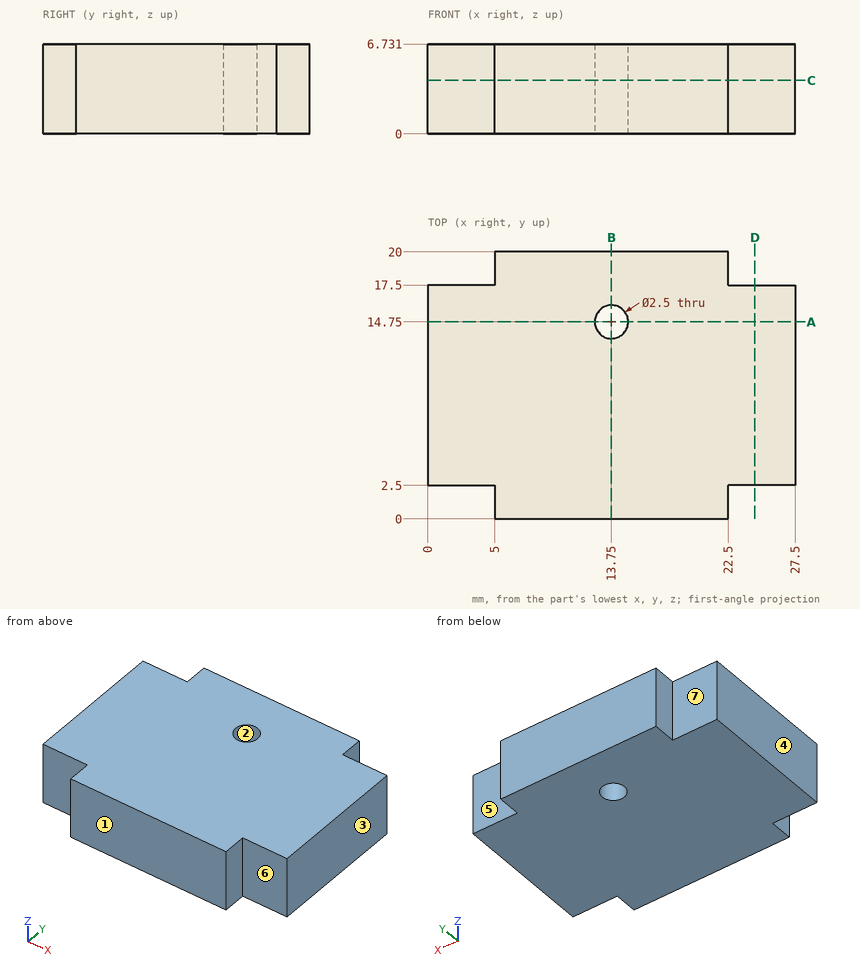
Geometry: see drawing. Coordinates: mm, zero at the bounding-box minimum. A direction names the side the tool comes from. Give positions to 0.01 mm unless a question says otherwise; leave off trailing zeros. Order: outer loops, then holes, each group sorted by start corner. A loop starts at its lowest first (then second) coordinate and runs counter-clockwise, first axis right, second up. Notation, with made-up numbers: M 86.5,-20.75 L 126.5,-20.75 A25 cw 126.5,15.25 Z; hole C -32.5,60.25 d10. An arc over 180 degrees is marked long. Answer as a JSON object with one key per item and string values.
1. First-contact query: P1, Ø1.5, axis at x = 24, z = 4, coming from the -Y side; P2, Ø2.5, axis at x = 1.5, z = 3.5, coming from the +Y side; P3, Ø2, axis at y = 19, z = 2.5, coming from the -X side; P4, Ø2, axis at x = 13.75, y = 14.75, coming from the -Z side. Flat tips, straight axial feed; report the tip coordinate or a pass-through.
Result sheet:
{"P1": "y = 2.5", "P2": "y = 17.5", "P3": "x = 5", "P4": "through"}
2. Reachability of the marked faces 5, 6 and 7 from +Z, -Z, +X, -X, +Y, -Y: full face, straight path, thin tool, end or side. Return the list, or none.
Result sheet:
{"face 5": "+Z, -Z, +X, +Y", "face 6": "+Z, -Z, +X, -Y", "face 7": "+Z, -Z, -X, +Y"}
3. Ray query, line 1 (Y direction, x = 13.75, z = 2.5); line 2 (Y direction, x = 14.75, z = 2.5); line 3 (X direction, y = 1.5, z = 3.75). Return the intervals inside material, ascending. Write a range as [from, to].
Result sheet:
{"line 1": "[0, 13.5], [16, 20]", "line 2": "[0, 14], [15.5, 20]", "line 3": "[5, 22.5]"}
4. Pull-direction query (X, two-part tool) for the marked faces 1, 2, 3 and 4; classes: +X half, -X half, draft (parallel to the pull), parting line (faces both ways), or undercut.
Result sheet:
{"face 1": "draft", "face 2": "undercut", "face 3": "+X half", "face 4": "-X half"}
5. Cut plane A-A, the plane y = 14.75. Output: boundary loops of the cut face in (x, z).
Result sheet:
{"outline": "M 0,0 L 12.5,0 L 12.5,6.73 L 0,6.73 Z; M 15,0 L 27.5,0 L 27.5,6.73 L 15,6.73 Z"}
6. Cut plane C-C, the plane z = 4. Output: boundary loops of the cut face in (x, y), and give its area (3 significant figures).
Result sheet:
{"outline": "M 0,2.5 L 5,2.5 L 5,0 L 22.5,0 L 22.5,2.5 L 27.5,2.5 L 27.5,17.5 L 22.5,17.5 L 22.5,20 L 5,20 L 5,17.5 L 0,17.5 Z; hole C 13.75,14.75 d2.5", "area": "495 mm²"}
7. Cut plane B-B, the plane x = 13.75. Output: boundary loops of the cut face in (y, z).
Result sheet:
{"outline": "M 0,0 L 13.5,0 L 13.5,6.73 L 0,6.73 Z; M 16,0 L 20,0 L 20,6.73 L 16,6.73 Z"}
8. Cut plane D-D, the plane x = 24.5. Output: boundary loops of the cut face in (y, z), and give its area (3 significant figures).
Result sheet:
{"outline": "M 2.5,0 L 17.5,0 L 17.5,6.73 L 2.5,6.73 Z", "area": "101 mm²"}
